from build123d import *

# Parameters (mm, degrees)
BOSS_EXTRUDE1_DEPTH = 3
CHAMFER1_SIZE       = 1


with BuildPart() as part:
    # Sketch1 → Boss-Extrude1 (new body)
    with BuildSketch(Plane(origin=(0, 0, 0), x_dir=(1, 0, 0), z_dir=(0, 1, 0))):
        Polygon((-170, -97.5), (-170, -22.5), (-150, -22.5), (-150, 27.5), (-170, 27.5), (-170, 97.5), (170, 97.5), (170, 27.5), (150, 27.5), (150, -22.5), (170, -22.5), (170, -97.5), align=None)
    extrude(amount=BOSS_EXTRUDE1_DEPTH)

    # Chamfer1
    chamfer1_edges = [part.edges().sort_by_distance(p)[0] for p in [
        (-170, 1.5, 97.5),
        (170, 1.5, 97.5),
    ]]
    chamfer(chamfer1_edges, length=CHAMFER1_SIZE)


solid = part.part
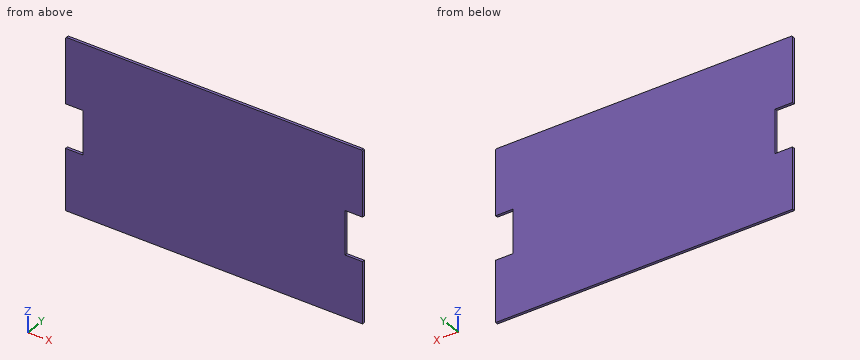
Could you check a few things on this model? Use its own coordinates, in mm. Round coordinates to 2 decimals unless told otherwise and drop trailing zeros. Order: outer loops, then holes, each group sorted by start corner. A loop starts at its lowest first (then second) coordinate and runs counter-clockwise, first axis right, second up.
Q1. I'm going to push flat-ended pins straight in: P1, Ø1.5, axis at y = 1.5, z = 2.5, coming from the -X side; P2, Ø1.5, axis at x = 94, z = -30.5, coming from the -Y side. Where does each tip first touch, or does it pass through?
Geometry says:
P1: stops at x = -150
P2: stops at y = 0
Q2. Imagine slicing it at A-A, the plane y = 1.2. List the corners of the cut face in (x, z) for me.
Geometry says:
outline: (-170, -97.5) - (170, -97.5) - (170, -27.5) - (150, -27.5) - (150, 22.5) - (170, 22.5) - (170, 96.5) - (169, 97.5) - (-169, 97.5) - (-170, 96.5) - (-170, 22.5) - (-150, 22.5) - (-150, -27.5) - (-170, -27.5) - close
Q3. Imagine slicing it at B-B, the plane z = -5.5. List the corners of the cut face in (x, y) for me, then the cut area to 3 significant figures.
Geometry says:
outline: (-150, 0) - (150, 0) - (150, 3) - (-150, 3) - close
area: 900 mm2
Q4. Please list where these lines run through material, in increasing order: probe 1 along Z at (x, y) = (151, 2.85); probe 2 along X at (y, z) = (1.05, 4).
Geometry says:
probe 1: z = -97.5 to -27.5, 22.5 to 97.5
probe 2: x = -150 to 150
